Could you check a few things on this model? Use its own coordinates, in mm. A direction names the side the tool comes from. Round coordinates to 2 decimals unless told otherwise and drop trailing zeros. Order: outer loops, then holes, each group sorted by start corner. A loop starts at its lowest first (then second) coordinate and runs counter-clockwise, first axis right, second up. Notation, with made-up numbers: (-17, -39) -> (29, -39) arc R13 ccw to (29, -18) -> close; hole circle Ø6 at (75, 7). An arc over 180 degrees is marked (long way). Put each result on its own line as item: value. Start each with the question number.
from build123d import *

# Parameters (mm, degrees)
BOSS_EXTRUDE1_DEPTH     = 10
CUT_EXTRUDE1_DEPTH      = 36.756118358
CUT_EXTRUDE1_DEPTH_BACK = 36.756118358
SKETCH2_R               = 1.75
SKETCH3_R               = 1.65
CUT_EXTRUDE2_DEPTH      = 27.96757312
FILLET1_R               = 3


with BuildPart() as part:
    # Sketch1 → Boss-Extrude1 (new body)
    with BuildSketch(Plane(origin=(0, 0, 0), x_dir=(1, 0, 0), z_dir=(0, 1, 0))):
        Polygon((-22.5, -7.5), (22.5, -7.5), (22.5, -3.5), (11, -3.5), (11, 7.5), (7, 7.5), (7, -3.5), (-7, -3.5), (-7, 7.5), (-11, 7.5), (-11, -3.5), (-22.5, -3.5), align=None)
    extrude(amount=BOSS_EXTRUDE1_DEPTH)

    # Sketch2 → Cut-Extrude1 (cut, two sides: drawn at the far end of the back side and taken through both)
    with BuildSketch(Plane.ZY.offset(11).offset(-CUT_EXTRUDE1_DEPTH_BACK)):
        with BuildLine():
            Line((-7.5, 10), (-7.5, 5))
            ThreePointArc((-7.5, 5), (-6.035533906, 8.535533906), (-2.5, 10))
            Line((-2.5, 10), (-7.5, 10))
        make_face()
        with BuildLine():
            Line((-7.5, 0), (-2.5, 0))
            ThreePointArc((-2.5, 0), (-6.035533906, 1.464466094), (-7.5, 5))
            Line((-7.5, 5), (-7.5, 0))
        make_face()
        with Locations((-2.5, 5)):
            Circle(SKETCH2_R)
    extrude(amount=CUT_EXTRUDE1_DEPTH + CUT_EXTRUDE1_DEPTH_BACK, mode=Mode.SUBTRACT)

    # Sketch3 → Cut-Extrude2 (cut, through all)
    with BuildSketch(Plane(origin=(0, 0, 3.5), x_dir=(-1, 0, 0), z_dir=(0, 0, -1))):
        with Locations((16.75, 5)):
            Circle(SKETCH3_R)
        with Locations(Location((-16.75, 5, 0), (0, 0, 180))):
            Circle(SKETCH3_R)
    extrude(amount=-CUT_EXTRUDE2_DEPTH, mode=Mode.SUBTRACT)

    # Fillet1
    fillet1_edges = [part.edges().sort_by_distance(p)[0] for p in [
        (22.5, 0, 5.5),
        (-22.5, 0, 5.5),
        (-11, 5, 3.5),
        (-7, 5, 3.5),
        (7, 5, 3.5),
        (11, 5, 3.5),
        (-22.5, 10, 5.5),
        (22.5, 10, 5.5),
    ]]
    fillet(fillet1_edges, radius=FILLET1_R)


solid = part.part
1. I need wall thicknesses on L1, parallel to Z at x = 7.95, y = 5; L2, parallel to X at y = 8, z = 0.75; L3, parallel to Y at x = -10.05, z = -2.5. Which ranges of each line are inside material? Lowest first, please.
2. For pin 1 Ø5 at (y, z) = (7.5, 4) entering from +X; pin 2 Ø2 at (y, z) = (5, -2.5) entering from +X; pin 3 Ø2.5 at (y, z) = (2.5, -3) entering from +X; pin 4 Ø2.5 at (y, z) = (7.5, -3.5) entering from -X, each with a flat end and sliding along its axis, tell me the tip position at first contact or that it passes through.
3. If we section it at B-B, the plane x = -16.75: Please give me the cut outline in (y, z), then the cut area to 3 significant figures.
4. If we section it at D-D, the plane x = 8: Please give me the cut outline in (y, z).
5. Which directions (+Z, -Z, +X, -X, +Y, -Y) give clear straight access to the entire face, cutting with the end or side of a thin tool? Please do faces 1 (the face through (0, 5, 3.5)), 2 (the face through (-11, 4.9, -4.4)), 3 (the face through (-22.5, 5, 5)).
6. If we section it at C-C, the plane z = 0: Please give me the cut outline in (x, y).
7. If we section it at A-A, the plane z = 6.5: Please give me the cut outline in (x, y), then the cut area to 3 significant figures.
8. Thinking about a two-plate mould opening in X: for faces 4 (the face through (7, 4.9, -4.4)), 5 (the face through (21.6, 0.86, 5.47)), 6 (the face through (-21.64, 0.9, 5.53)), 7 (the face through (19, 5, 3.5)), which applies, +X half, -X half, draft (parallel to the pull), parting line (faces both ways), or undercut?
Results below:
1. L1: -7.5 to -4.25, -0.75 to 7.5
1. L2: -11.01 to -6.99, 6.99 to 11.01
1. L3: 0 to 3.25, 6.75 to 10
2. pin 1: x = 22.5
2. pin 2: through
2. pin 3: x = 11
2. pin 4: x = -11
3. outline: (0, 3.5) -> (3.35, 3.5) -> (3.35, 7.5) -> (0, 7.5) -> close; (6.65, 3.5) -> (10, 3.5) -> (10, 7.5) -> (6.65, 7.5) -> close
3. area: 26.8 mm2
4. outline: (0, -2.5) arc R5 ccw to (10, -2.5) -> (10, 7.5) -> (0, 7.5) -> close; hole circle Ø3.5 at (5, -2.5)
5. face 1: -Z, +Y, -Y
5. face 2: -Z, -X, +Y, -Y
5. face 3: +Z, -Z, -X, +Y, -Y
6. outline: (-11, 0) -> (-7, 0) -> (-7, 10) -> (-11, 10) -> close; (7, 0) -> (11, 0) -> (11, 10) -> (7, 10) -> close
7. outline: (-22.5, 3) arc R3 ccw to (-19.5, 0) -> (19.5, 0) arc R3 ccw to (22.5, 3) -> (22.5, 7) arc R3 ccw to (19.5, 10) -> (-19.5, 10) arc R3 ccw to (-22.5, 7) -> close; hole circle Ø3.3 at (-16.75, 5); hole circle Ø3.3 at (16.75, 5)
7. area: 425 mm2
8. face 4: undercut
8. face 5: +X half
8. face 6: -X half
8. face 7: draft
